Could you check a few things on this model? Use its own coordinates, in mm. A direction names the side the tool comes from. Round coordinates to 2 decimals unless told otherwise and drop trailing zeros. Loops run counter-clockwise (first coordinate to the right, second up) from the corner with the lowest first, then second, coordinate; pieces in that order, holes last.
from build123d import *

# Parameters (mm, degrees)
F0_W     = 65
F0_H     = 95
F1_DEPTH = 20
F2_W     = 62
F2_H     = 92
F3_DEPTH = 20
F5_W     = 10
F5_H     = 2
F4_W     = 10
F4_H     = 20


with BuildPart() as f1:
    # F0 (on Top) → F1 (new body)
    with BuildSketch(Plane.XY):
        Rectangle(F0_W, F0_H)
    extrude(amount=F1_DEPTH)

    # F2 (on face) → F3 (cut, through all)
    with BuildSketch(Plane.XY.offset(20)):
        Rectangle(F2_W, F2_H)
    extrude(amount=-F3_DEPTH, mode=Mode.SUBTRACT)

    # F5 (on face) → F6 section 0
    with BuildSketch(Plane(origin=(0, -46, 0), x_dir=(-1, 0, 0), z_dir=(0, 1, 0))):
        with Locations((0, 1)):
            Rectangle(F5_W, F5_H)
    # F4 (on face) → F6 section 1
    with BuildSketch(Plane.XZ.offset(-46)):
        with Locations((0, 10)):
            Rectangle(F4_W, F4_H)
    loft()


solid = f1.part
Item 1: If we section it at C-C, the plane y = -32: Count the separate pieces of the cut face and the enclosed holes in it, then the cut area to 3 significant figures.
Results list:
separate pieces: 3
enclosed holes: 0
area: 107 mm2
Item 2: If I drill on line 1 along X through (y, z) = (-2.5, 1.5); line 2 along Y through (x, z) = (-16, 5); line 3 along X through (y, z) = (-13, 17.75), over which ranges is the centre line in solid material (lowest first)?
Results list:
line 1: x = -32.5 to -31, -5 to 5, 31 to 32.5
line 2: y = -47.5 to -46, 46 to 47.5
line 3: x = -32.5 to -31, 31 to 32.5
Item 3: We'd pull the mould along X, two halves only. Please class faces 1 (the flat face through (32.5, -1, 10)), 2 (the flat face through (0, 47.5, 10)), 3 (the flat face through (18, 46, 10)): released by +X, released by -X, zero draft, split by the parting line, or undercut.
Results list:
face 1: released by +X
face 2: zero draft
face 3: undercut
Item 4: If we section it at B-B, the plane x = -3.5: Please give me the cut outline in (y, z), then the cut area to 3 significant figures.
Results list:
outline: (-47.5, 0) - (47.5, 0) - (47.5, 20) - (46, 20) - (-46, 2) - (-46, 20) - (-47.5, 20) - close
area: 1,070 mm2
Item 5: For faces 4 (the flat face through (-31, -1, 10)), 5 (the flat face through (-3, 0, 0)), 6 (the flat face through (-0.07, 0.644, 11.126)), which set-ups out of +Z, -Z, +X, -X, +Y, -Y let a thin tool reach every point of the face, with its end or its side?
Results list:
face 4: +Z, -Z
face 5: -Z, +X, -X, +Y, -Y
face 6: +Z
Item 6: If we section it at A-A, the plane x = 9.5: Please give me the cut outline in (y, z), then the cut area to 3 significant figures.
Results list:
outline: (-47.5, 0) - (-46, 0) - (-46, 20) - (-47.5, 20) - close; (46, 0) - (47.5, 0) - (47.5, 20) - (46, 20) - close
area: 60.0 mm2
